Model file for the job. Use its own axes, mm. Face numbers are marked on the shaded views. A direction names the side the tool comes from. Round coordinates to 2 decimals unless told otherwise and drop trailing zeros. Loops run counter-clockwise (first coordinate to the right, second up) from the corner with the lowest first, then second, coordinate; pieces in that order, holes last.
from build123d import *

# Parameters (mm, degrees)
F0_W          = 101.6
F0_H          = 101.6
F1_DEPTH      = 50.8
F3_DEPTH      = 50.801
F5_DEPTH      = 42.6892808993
F5_DEPTH_BACK = 42.6892808993
F7_DEPTH      = 42.6892808993
F7_DEPTH_BACK = 42.6892808993
F9_DEPTH      = 25.4
F9_DEPTH_BACK = 25.4
F10_R         = 12.7
F10_R_2       = 10.16
F11_DEPTH     = 36.068
F12_R         = 10.16
F13_DEPTH     = 25.4
F14_R         = 10.16
F15_DEPTH     = 5.334
F16_W         = 3.048
F16_H         = 14.3684097937
F17_DEPTH     = 12.7
F18_W         = 14.3684097937
F18_H         = 3.81
F19_DEPTH     = 5.334


with BuildPart() as f1:
    # F0 (on Top) → F1 (new body)
    with BuildSketch(Plane.XY):
        Rectangle(F0_W, F0_H)
    extrude(amount=F1_DEPTH)

    # F2 (on face) → F3 (cut, through all)
    with BuildSketch(Plane.XY.offset(50.8)):
        Polygon((-1.5875, 50.8), (-50.8, 50.8), (-50.8, 1.5875), (-50.8, -1.5875), (-50.8, -50.8), (-1.5875, -50.8), (1.5875, -50.8), (50.8, -50.8), (50.8, -1.5875), (50.8, 1.5875), (50.8, 50.8), (1.5875, 50.8), align=None)
        Polygon((-42.6882808993, -1.5875), (-42.6882808993, 1.5875), (-1.5875, 1.5875), (-1.5875, 42.6882808993), (1.5875, 42.6882808993), (1.5875, 1.5875), (42.6882808993, 1.5875), (42.6882808993, -1.5875), (1.5875, -1.5875), (1.5875, -42.6882808993), (-1.5875, -42.6882808993), (-1.5875, -1.5875), align=None, mode=Mode.SUBTRACT)
    extrude(amount=-F3_DEPTH, mode=Mode.SUBTRACT)

    # F4 (on Front) → F5 (cut, two sides)
    with BuildSketch(Plane.XZ) as f5_sk:
        Polygon((0, 44.45), (42.6882808993, 0), (42.6882808993, 50.8), (-42.6882808993, 50.8), (-42.6882808993, 0), align=None)
    extrude(amount=-F5_DEPTH, mode=Mode.SUBTRACT)
    extrude(f5_sk.sketch, amount=F5_DEPTH_BACK, mode=Mode.SUBTRACT)

    # F6 (on Right) → F7 (cut, two sides)
    with BuildSketch(Plane.YZ) as f7_sk:
        Polygon((-42.6882808993, 50.8), (-42.6882808993, 0), (0, 44.45), (42.6882808993, 0), (42.6882808993, 50.8), align=None)
    extrude(amount=-F7_DEPTH, mode=Mode.SUBTRACT)
    extrude(f7_sk.sketch, amount=F7_DEPTH_BACK, mode=Mode.SUBTRACT)

    # F8 (on Front) → F9 (cut, two sides)
    with BuildSketch(Plane.XZ) as f9_sk:
        Polygon((0, 64.3248185515), (-9.6034230664, 42.5812155008), (15.0393228978, 42.5812155008), align=None)
    extrude(amount=-F9_DEPTH, mode=Mode.SUBTRACT)
    extrude(f9_sk.sketch, amount=F9_DEPTH_BACK, mode=Mode.SUBTRACT)

    # F10 (on face) → F11 (cut)
    with BuildSketch(Plane.XY.offset(42.5812155008)):
        Circle(F10_R)
        Circle(F10_R_2, mode=Mode.SUBTRACT)
    extrude(amount=-F11_DEPTH, mode=Mode.SUBTRACT)

    # F12 (on face) → F13 (cut)
    with BuildSketch(Plane.XY.offset(42.5812155008)):
        Circle(F12_R)
    extrude(amount=-F13_DEPTH, mode=Mode.SUBTRACT)

    # F14 (on Top) → F15 (join)
    with BuildSketch(Plane.XY):
        Circle(F14_R)
    extrude(amount=F15_DEPTH)

    # F16 (on face) → F17 (join)
    with BuildSketch(Plane(origin=(0, 0, 0), x_dir=(1, 0, 0), z_dir=(0, 0, -1))):
        with Locations((5.6602048969, 0)):
            Rectangle(F16_W, F16_H)
    extrude(amount=F17_DEPTH)

    # F18 (on face) → F19 (join)
    with BuildSketch(Plane(origin=(4.1362048969, 0, 0), x_dir=(0, -1, 0), z_dir=(-1, 0, 0))):
        with Locations((0, -10.795)):
            Rectangle(F18_W, F18_H)
    extrude(amount=F19_DEPTH)


solid = f1.part
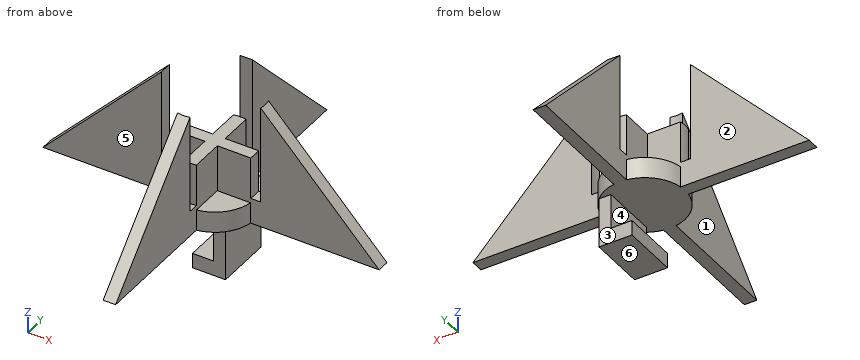
Q1. Slice it at D-D on z = 3. Give the cut face in (x, y), plus the area to 3 significant figures.
Q2. Slice it at C-C on y = 21. Give the cut face in (x, z), plus the area to 3 significant figures.
Q3. Tool access for the marked faces 1, 2 and 3: list every direction of +Z, -Z, +X, -X, +Y, -Y with a clear straight run to the whole face (end or side of a thin tool).
Q4. Flat gauge pins, fed straight in: P1, Ø6, axis at x = 24.5, z = 14, coming from the -Y side; P2, Ø9.5, axis at x = -5, y = 5.5, coming from the +Z side; P3, Ø6, axis at y = 32.5, z = 4, coming from the -X side. Where does each tip first touch, or does it go through?
Q5. Slice it at B-B on x = -8. Give the cut face in (y, z).
Q6. Probe line 1 (Y direction, x = 21, z = 2); line 2 (Z direction, x = 0.5, y = 18.5). List the from-to ranges inside material, lowest first.
Q7. Slice it at A-A on z = 24.5. Give the cut face in (x, y), plus the area to 3 significant figures.
Q8. Pull direction Z, two halves, no side cores. Call the marked faces 4, 5 and 6: pulls with the +Z half, pulls with the -Z half, needs draft (parallel to the pull), parting line crosses it, or undercut.
Reply:
1. outline: (-39.81, -1.59) - (-10.04, -1.59) arc R10.16 ccw to (-1.59, -10.04) - (-1.59, -39.81) - (1.59, -39.81) - (1.59, -10.04) arc R10.16 ccw to (10.04, -1.59) - (39.81, -1.59) - (39.81, 1.59) - (10.04, 1.59) arc R10.16 ccw to (1.59, 10.04) - (1.59, 39.81) - (-1.59, 39.81) - (-1.59, 10.04) arc R10.16 ccw to (-10.04, 1.59) - (-39.81, 1.59) - close
1. area: 701 mm2
2. outline: (-1.59, 0) - (1.59, 0) - (1.59, 22.58) - (-1.59, 22.58) - close
2. area: 71.7 mm2
3. face 1: +Z, -X, -Y
3. face 2: +Z, -X, +Y
3. face 3: -Z, +X, -X, +Y
4. P1: stops at y = -1.59
4. P2: stops at z = 17.18
4. P3: stops at x = -1.59
5. outline: (-6.26, 0) - (6.26, 0) - (6.26, 5.33) - (1.59, 5.33) - (1.59, 17.18) - (-1.59, 17.18) - (-1.59, 5.33) - (-6.26, 5.33) - close
6. line 1: y = -1.59 to 1.59
6. line 2: z = 0 to 25.19
7. outline: (-19.16, -1.59) - (-12.6, -1.59) arc R12.7 cw to (-12.6, 1.59) - (-19.16, 1.59) - close; (-1.59, -19.16) - (1.59, -19.16) - (1.59, -12.6) arc R12.7 cw to (-1.59, -12.6) - close; (-1.59, 12.6) arc R12.7 cw to (1.59, 12.6) - (1.59, 19.16) - (-1.59, 19.16) - close; (12.6, -1.59) - (19.16, -1.59) - (19.16, 1.59) - (12.6, 1.59) arc R12.7 cw to start
7. area: 82.5 mm2
8. face 4: undercut
8. face 5: needs draft
8. face 6: pulls with the -Z half
